```python
from build123d import *

# Parameters (mm, degrees)
BOSS_EXTRUDE1_DEPTH     = 80
CUT_EXTRUDE1_DEPTH      = 227.715680975
CUT_EXTRUDE1_DEPTH_BACK = 227.715680975
SKETCH2_R               = 4
SKETCH5_W               = 15
SKETCH5_H               = 15
BOSS_EXTRUDE2_DEPTH     = 90
FILLET1_R               = 30


with BuildPart() as part:
    # Sketch1 → Boss-Extrude1 (new body)
    with BuildSketch(Plane(origin=(0, 0, 0), x_dir=(1, 0, 0), z_dir=(0, 1, 0))):
        Polygon((-150, 150), (150, 150), (150, -150), (94, -94), (94, 147), (-94, 147), (-94, -94), (-150, -150), align=None)
        Polygon((-147, 147), (-97, 147), (-97, -92.757359313), (-147, -142.757359313), align=None, mode=Mode.SUBTRACT)
        Polygon((147, 147), (147, -142.757359313), (97, -92.757359313), (97, 147), align=None, mode=Mode.SUBTRACT)
    extrude(amount=BOSS_EXTRUDE1_DEPTH)

    # Sketch2 → Cut-Extrude1 (cut, two sides: drawn at the far end of the back side and taken through both)
    with BuildSketch(Plane(origin=(0, 0, 0), x_dir=(0, 0, -1), z_dir=(1, 0, 0)).offset(-CUT_EXTRUDE1_DEPTH_BACK)):
        with Locations((115, 28)):
            Circle(SKETCH2_R)
        with Locations((-5, 28)):
            Circle(SKETCH2_R)
    extrude(amount=CUT_EXTRUDE1_DEPTH + CUT_EXTRUDE1_DEPTH_BACK, mode=Mode.SUBTRACT)

    # Sketch5 → Boss-Extrude2 (add)
    with BuildSketch(Plane(origin=(0, 0, 0), x_dir=(1, 0, 0), z_dir=(0, 1, 0))):
        Polygon((-150, -127), (-135, -127), (-135, -135), (-150, -150), (-150, -140.427238406), align=None)
        Polygon((150, -150), (135, -135), (135, -127), (150, -127), (150, -140.427238406), align=None)
        with Locations((142.5, 142.5)):
            Rectangle(SKETCH5_W, SKETCH5_H)
        with Locations((-142.5, 142.5)):
            Rectangle(SKETCH5_W, SKETCH5_H)
    extrude(amount=BOSS_EXTRUDE2_DEPTH)

    # Fillet1
    fillet1_edges = [part.edges().sort_by_distance(p)[0] for p in [
        (94, 40, 94),
        (-94, 40, 94),
    ]]
    fillet(fillet1_edges, radius=FILLET1_R)


solid = part.part
```
Work out the finished part from the listing and answer in its coordinate system (mm). A direction names the side the tool comes from. Coordinates: 2 decimals unless noted, no trailing zeros. Order: outer loops, then holes, each group sorted by start corner. A loop starts at its lowest first (then second) coordinate and runs counter-clockwise, first axis right, second up. Notation, with made-up numbers: (-12, 48.5) - (22, 48.5) arc R8 cw to (22, 54.5) - close; hole circle Ø4 at (37, 89). An arc over 180 degrees is marked (long way). Answer as a JSON object with one key per item and string values.
1. Find section B-B on z = -115. Count the separate pieces of the cut face and the enclosed holes in it, plus the area to 3 significant figures.
Output values:
{"separate pieces": "8", "enclosed holes": "0", "area": "864 mm²"}
2. Find section C-C on y = 14. Determine the outline of the cut face in (x, z).
Output values:
{"outline": "(-150, -150) - (150, -150) - (150, 150) - (102.79, 102.79) arc R30 ccw to (94, 81.57) - (94, -147) - (-94, -147) - (-94, 81.57) arc R30 ccw to (-102.79, 102.79) - (-150, 150) - close; hole (-147, -135) - (-135, -135) - (-135, -147) - (-97, -147) - (-97, 92.76) - (-135, 130.76) - (-135, 127) - (-147, 127) - close; hole (97, -147) - (135, -147) - (135, -135) - (147, -135) - (147, 127) - (135, 127) - (135, 130.76) - (97, 92.76) - close"}
3. Consider line 1 (Z direction, x = -96.2, y = 28); line 2 (X direction, y = 14.5, z = 59.5); line 3 (X direction, y = 35, z = 135). Determine where each line is inside the solid, lowest interval first.
Output values:
{"line 1": "z = -150 to -119, -111 to 1, 9 to 92.85", "line 2": "x = -150 to -147, -97 to -94, 94 to 97, 147 to 150", "line 3": "x = -150 to -135, 135 to 150"}
4. Find section A-A on z = -83. Determine the outline of the cut face in (x, y).
Output values:
{"outline": "(-150, 0) - (-147, 0) - (-147, 80) - (-150, 80) - close; (-97, 0) - (-94, 0) - (-94, 80) - (-97, 80) - close; (94, 0) - (97, 0) - (97, 80) - (94, 80) - close; (147, 0) - (150, 0) - (150, 80) - (147, 80) - close"}
5. The mould has two halves that part along X. Classify faces 4 (the face through (148.479, 31.966, 5.521)), 5 (the face through (147, 39, -6)), 6 (the face through (150, 44, -2)): +X half, -X half, draft (parallel to the pull), parting line (faces both ways), or undercut.
Output values:
{"face 4": "draft", "face 5": "undercut", "face 6": "+X half"}
6. Each of these flat-tipped pins is pushed along its axis until it touches: P1, Ø7, axis at y = 28, z = 5, coming from the -X side; P2, Ø5, axis at x = -31.5, y = 37, coming from the +Z side; P3, Ø3.5, axis at x = 148, z = 40.5, coming from the +Y side; P4, Ø19, axis at x = -117, y = 33, coming from the +Z side. Where does it stop, or does it pass through?
Output values:
{"P1": "passes through", "P2": "stops at z = -147", "P3": "stops at y = 80", "P4": "stops at z = 126.5"}
7. A tool of negligible diameter and unlimited length cuts with its end or side. For faces 1 (the face through (-97, 39, -29)), 2 (the face through (-150, 44, 2)), 3 (the face through (127, 44, 127)), from which of +Z, -Z, +X, -X, +Y, -Y can it reach the whole face along a straight path? Write none if from no direction.
Output values:
{"face 1": "+Y, -Y", "face 2": "+Z, -Z, -X, +Y, -Y", "face 3": "+Z, +Y, -Y"}
8. Find section D-D on x = -107. Determine the outline of the cut face in (y, z).
Output values:
{"outline": "(0, -150) - (80, -150) - (80, -147) - (0, -147) - close; (0, 102.76) - (80, 102.76) - (80, 107) - (0, 107) - close"}
